Could you check a few things on this model? Use its own coordinates, in mm. Face numbers are marked on the shaded views. A direction names the side the tool comes from. Give positions to 0.01 mm unless a question says otherwise; leave off trailing zeros. Write each loop counter-clockwise with the first axis right and the second up, starting at its lowest first coordinate (ties: lowest second). Pieces come first, ordered by that corner, then holes. Notation, with made-up numbers: M 46,29.5 L 89,29.5 A13 ccw 89,47.5 Z; hole C 49.25,9.5 d4. An arc over 180 degrees is marked long. One line per item, written item: value.
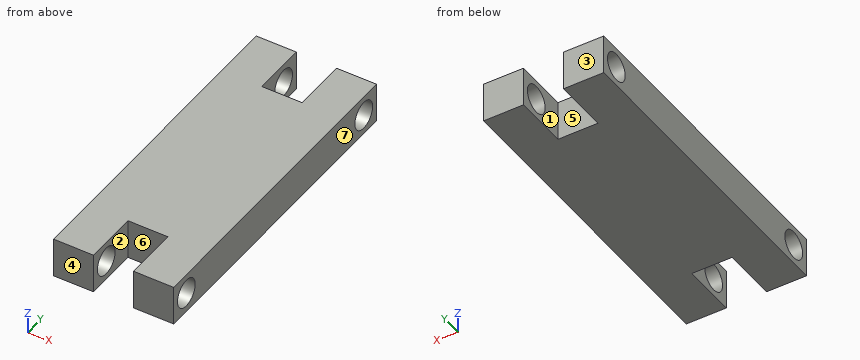
```python
from build123d import *

# Parameters (mm, degrees)
F1_DEPTH = 12.7
F2_R     = 4.445
F3_DEPTH = 38.1


with BuildPart() as f1:
    # F0 (on Top) → F1 (new body)
    with BuildSketch(Plane.XY):
        Polygon((12.7, 50.8), (0, 50.8), (0, -50.8), (12.7, -50.8), (12.7, -33.558697), (25.4, -33.558697), (25.4, -50.8), (38.1, -50.8), (38.1, 50.8), (25.4, 50.8), (25.4, 33.558697), (12.7, 33.558697), align=None)
    extrude(amount=F1_DEPTH)

    # F2 (on face) → F3 (cut, through all)
    with BuildSketch(Plane(origin=(0, 0, 0), x_dir=(0, -1, 0), z_dir=(-1, 0, 0))):
        with Locations((-44.45, 6.35)):
            Circle(F2_R)
        with Locations((44.45, 6.35)):
            Circle(F2_R)
    extrude(amount=-F3_DEPTH, mode=Mode.SUBTRACT)


solid = f1.part
```
1) I'm going to push flat-ended pins straight in: pin 1 (5 mm diameter, centred on x = 18.5, z = 5.5, fed in from +Y); pin 2 (2 mm diameter, centred on x = 15.5, y = -37.5, fed in from -Z). Where does each tip first touch, or does it pass through?
Outcome:
pin 1: stops at y = 33.56
pin 2: passes through
2) If we section it at A-A, the plane y = -34.5: Write out the boundary of the cut face in (x, z), then the cut area to 3 significant figures.
Outcome:
outline: M 0,0 L 12.7,0 L 12.7,12.7 L 0,12.7 Z; M 25.4,0 L 38.1,0 L 38.1,12.7 L 25.4,12.7 Z
area: 323 mm^2
3) On a 3-axis mill with a long thin cutter (end or side, diameter ignored), from which of +Z, -Z, +X, -X, +Y, -Y can I reach the whole of each face in a straight line? I mean the marked faces 1, 2 and 3. Say none if no direction works.
Outcome:
face 1: +Z, -Z, +Y
face 2: +Z, -Z, -Y
face 3: +Z, -Z, +X, -X, +Y
4) Please list where these lines run through material, in increasing order: L1, parallel to Z at x = 9.5, y = 44.45 (3 decimals); L2, parallel to X at y = -34.5, z = 3.5; L3, parallel to Y at x = 33, z = 3. Write a range as from..to.
Outcome:
L1: z = 0..1.905, 10.795..12.7
L2: x = 0..12.7, 25.4..38.1
L3: y = -50.8..-47.37, -41.53..41.53, 47.37..50.8
5) If we section it at B-B, the plane z = 6.35: Write out the boundary of the cut face in (x, y) (3 decimals), then the cut area to 3 significant figures.
Outcome:
outline: M 0,-50.8 L 12.7,-50.8 L 12.7,-48.895 L 0,-48.895 Z; M 0,-40.005 L 12.7,-40.005 L 12.7,-33.559 L 25.4,-33.559 L 25.4,-40.005 L 38.1,-40.005 L 38.1,40.005 L 25.4,40.005 L 25.4,33.559 L 12.7,33.559 L 12.7,40.005 L 0,40.005 Z; M 0,48.895 L 12.7,48.895 L 12.7,50.8 L 0,50.8 Z; M 25.4,-50.8 L 38.1,-50.8 L 38.1,-48.895 L 25.4,-48.895 Z; M 25.4,48.895 L 38.1,48.895 L 38.1,50.8 L 25.4,50.8 Z
area: 2,980 mm^2
6) If we section it at C-C, the plane x = 26.5: Write out the boundary of the cut face in (y, z) (3 decimals).
Outcome:
outline: M -50.8,0 L 50.8,0 L 50.8,12.7 L -50.8,12.7 Z; hole C -44.45,6.35 d8.89; hole C 44.45,6.35 d8.89
7) We'd pull the mould along X, two halves only. Please class the marked faces 4, 5, 6 and 7: pulls with the +X half, pulls with the -X half, needs draft (parallel to the pull), parting line crosses it, or undercut.
Outcome:
face 4: needs draft
face 5: undercut
face 6: undercut
face 7: pulls with the +X half
8) If we section it at D-D, the plane y = 43: Write out the boundary of the cut face in (x, z).
Outcome:
outline: M 0,0 L 12.7,0 L 12.7,2.15 L 0,2.15 Z; M 0,10.55 L 12.7,10.55 L 12.7,12.7 L 0,12.7 Z; M 25.4,0 L 38.1,0 L 38.1,2.15 L 25.4,2.15 Z; M 25.4,10.55 L 38.1,10.55 L 38.1,12.7 L 25.4,12.7 Z
